```python
from build123d import *

# Parameters (mm, degrees)
F0_W     = 80
F0_H     = 15
F0_R     = 2.8
F1_DEPTH = 7.5
F2_SIZE  = 4
F3_SIZE  = 0.5
F5_D     = 2.5


with BuildPart() as f1:
    # F0 (on Top) → F1 (new body, symmetric)
    with BuildSketch(Plane.XY):
        with Locations((30, 0)):
            Rectangle(F0_W, F0_H)
        Circle(F0_R, mode=Mode.SUBTRACT)
        with Locations((20, 0)):
            Circle(F0_R, mode=Mode.SUBTRACT)
        with Locations((40, 0)):
            Circle(F0_R, mode=Mode.SUBTRACT)
        with Locations((60, 0)):
            Circle(F0_R, mode=Mode.SUBTRACT)
    extrude(amount=F1_DEPTH, both=True)

    # F2
    f2_edges = [f1.edges().sort_by_distance(p)[0] for p in [
        (-2.8, 0, 7.5),
        (17.2, 0, 7.5),
        (37.2, 0, 7.5),
        (57.2, 0, 7.5),
    ]]
    chamfer(f2_edges, length=F2_SIZE)

    # F3
    f3_edges = [f1.edges().sort_by_distance(p)[0] for p in [
        (57.2, 0, -7.5),
        (37.2, 0, -7.5),
        (17.2, 0, -7.5),
        (-2.8, 0, -7.5),
    ]]
    chamfer(f3_edges, length=F3_SIZE)

    # F5 (through all)
    with Locations(Plane(origin=(0, 7.5, 0), x_dir=(-1, 0, 0), z_dir=(0, 1, 0))):
        with Locations((-60, 0), (-40, 0), (-20, 0), (0, 0)):
            Hole(F5_D / 2)


solid = f1.part
```
Can you work these out from the model? Positions are in its coordinate system, mm. Coordinates: 2 decimals unless noted, no trailing zeros. Loops run counter-clockwise (first coordinate to the right, second up) from the corner with the lowest first, then second, coordinate; pieces in that order, holes last. Notation, with made-up numbers: (64.5, -14) - (73.5, -14) arc R36 cw to (73.5, 21) - close; hole circle Ø7 at (-11.75, 45.5). An arc over 180 degrees is marked (long way). Use a Markdown table: item, result.
Item 1: I want a section at A-A on x = 20. Please give me the cut outline in (y, z), and give its area (3 significant figures).
Numbers:
| item | result |
|---|---|
| outline | (-7.5, -7.5) - (-3.3, -7.5) - (-2.8, -7) - (-2.8, -1.25) - (-7.5, -1.25) - close; (-7.5, 1.25) - (-2.8, 1.25) - (-2.8, 3.5) - (-6.8, 7.5) - (-7.5, 7.5) - close; (2.8, -7) - (3.3, -7.5) - (7.5, -7.5) - (7.5, -1.25) - (2.8, -1.25) - close; (2.8, 1.25) - (7.5, 1.25) - (7.5, 7.5) - (6.8, 7.5) - (2.8, 3.5) - close |
| area | 101 mm2 |
Item 2: I want a section at C-C on y = 4.25. Give the number of separate pieces and of enclosed holes in the cut face, and give its area (3 significant figures).
Numbers:
| item | result |
|---|---|
| separate pieces | 1 |
| enclosed holes | 4 |
| area | 1,110 mm2 |
Item 3: Will these pins go through, and if not, where does the flat tip stop? pin 1 (7.5 mm diameter, centred on x = 0, y = 0, fed in from +Z); pin 2 (9 mm diameter, centred on x = 40, y = 0, fed in from +Z); pin 3 (3 mm diameter, centred on x = 40, z = 0, fed in from -Y).
Numbers:
| item | result |
|---|---|
| pin 1 | stops at z = 4.45 |
| pin 2 | stops at z = 5.2 |
| pin 3 | stops at y = -7.5 |
Item 4: We'd pull the mould along Z, two halves only. Please class faces 1 (the face through (29, 7.5, 0)), 2 (the face through (61.19, -5.04, 0.38)), 3 (the face through (37.6, -1.8, 3.7)): released by +Z, released by -Z, zero draft, split by the parting line, or undercut.
Numbers:
| item | result |
|---|---|
| face 1 | zero draft |
| face 2 | undercut |
| face 3 | released by +Z |
Item 5: If I drill on probe 1 along X at (y, z) = (3.85, 0); probe 2 along X at (y, z) = (2.5, 0); probe 3 along Z at (x, y) = (60, 4.75), over which ranges is the centre line in solid material (lowest first)? Write a range as from..to.
Numbers:
| item | result |
|---|---|
| probe 1 | x = -10..-1.25, 1.25..18.75, 21.25..38.75, 41.25..58.75, 61.25..70 |
| probe 2 | x = -10..-1.26, 1.26..18.74, 21.26..38.74, 41.26..58.74, 61.26..70 |
| probe 3 | z = -7.5..-1.25, 1.25..5.45 |
Item 6: I want a section at B-B on z = -5. Please give me the cut outline in (x, y).
Numbers:
| item | result |
|---|---|
| outline | (-10, -7.5) - (70, -7.5) - (70, 7.5) - (-10, 7.5) - close; hole circle Ø5.6 at (0, 0); hole circle Ø5.6 at (20, 0); hole circle Ø5.6 at (40, 0); hole circle Ø5.6 at (60, 0) |
